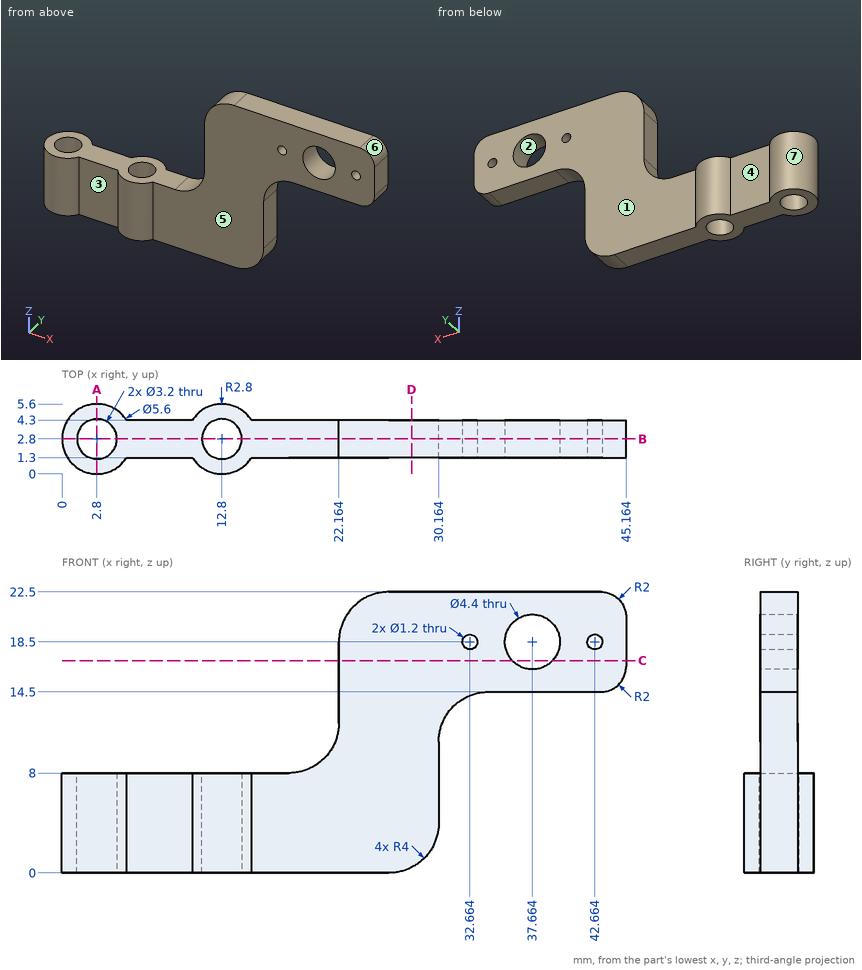
Geometry check sheet. Reference: drawing and pictorial views, mm from the part's lowest x, y, z. A direction names the side the tool comes from. Give positions to 0.01 mm unless a question says otherwise; leave off trailing zeros. Write each loop counter-clockwise with the first axis right and the second up, starting at its lowest first coordinate (ties: lowest second). Pieces come first, ordered by that corner, then holes.
Item 1: Cross-section at C-C (z = 17). Enter the section's corners in (x, y) (1 decimal).
Item 2: Scan lines: L1, parallel to X at y = 2.35, z = 18.5; L2, parallel to Y at x = 2.8, z = 3.5; L3, parallel to Y at x = 28.5, z = 4. Record each from-to range of solid material in increasing order.
Item 3: Gauge pin test, flat ends, axial feed: pin 1 (10 mm diameter, centred on x = 31.5, z = 3.5, fed in from +Y); pin 2 (4 mm diameter, centred on x = 7, z = 3, fed in from +Y); pin 3 (4 mm diameter, centred on x = 15, z = 6, fed in from +Y). Record the tip position at first contact, or that the pin passes through.
Item 4: Draft check along X on the marked faces 4, 5, 6 and 7. Enter one of: released by +X, released by -X, zero draft, split by the parting line, or undercut.
Item 5: Cross-section at D-D (x = 28). Enter the section's corners in (y, z).
Item 6: Access from +Z, -Z, +X, -X, +Y, -Y to the whole of each face (thin tool, end or side, straight path). Record for the marked faces 1, 2 and 3.
Item 7: Cross-section at A-A (x = 2.8). Enter the section's corners in (y, z).
Item 8: Cross-section at B-B (y = 2.8). Enter the section's corners in (x, z).
Report:
1. outline: (22.2, 1.3) - (36.1, 1.3) - (36.1, 4.3) - (22.2, 4.3) - close; (39.3, 1.3) - (45.2, 1.3) - (45.2, 4.3) - (39.3, 4.3) - close
2. L1: x = 22.16 to 32.06, 33.26 to 35.46, 39.86 to 42.06, 43.26 to 45.16
2. L2: y = 0 to 1.2, 4.4 to 5.6
2. L3: y = 1.3 to 4.3
3. pin 1: stops at y = 4.3
3. pin 2: stops at y = 4.53
3. pin 3: stops at y = 5.59
4. face 4: undercut
4. face 5: zero draft
4. face 6: released by +X
4. face 7: undercut
5. outline: (1.3, 0.45) - (4.3, 0.45) - (4.3, 22.5) - (1.3, 22.5) - close
6. face 1: +Z, -Z, +X, +Y
6. face 2: +Y, -Y
6. face 3: +Z, -Z, -Y
7. outline: (0, 0) - (1.2, 0) - (1.2, 8) - (0, 8) - close; (4.4, 0) - (5.6, 0) - (5.6, 8) - (4.4, 8) - close
8. outline: (0, 0) - (1.2, 0) - (1.2, 8) - (0, 8) - close; (4.4, 0) - (11.2, 0) - (11.2, 8) - (4.4, 8) - close; (14.4, 0) - (26.16, 0) arc R4 ccw to (30.16, 4) - (30.16, 10.5) arc R4 cw to (34.16, 14.5) - (43.16, 14.5) arc R2 ccw to (45.16, 16.5) - (45.16, 20.5) arc R2 ccw to (43.16, 22.5) - (26.16, 22.5) arc R4 ccw to (22.16, 18.5) - (22.16, 12) arc R4 cw to (18.16, 8) - (14.4, 8) - close; hole circle Ø1.2 at (32.66, 18.5); hole circle Ø4.4 at (37.66, 18.5); hole circle Ø1.2 at (42.66, 18.5)
